Answer from the drawing. Dimensions are ordinates in mm from the lowest x, y and z of the part. Coordinates: 2 decimals unless noted, no trailing zeros. Loops run counter-clockwise (first coordinate to the right, second up) from the corner with the lowest first, then second, coordinate; pieces in that order, holes last. Notation, with made-up numbers: (33, -11) -> (60, -11) arc R33 cw to (60, 18) -> close; hole circle Ø9 at (-27.75, 38.5). An arc over 180 degrees is marked (long way). Use a Markdown table: item, result.
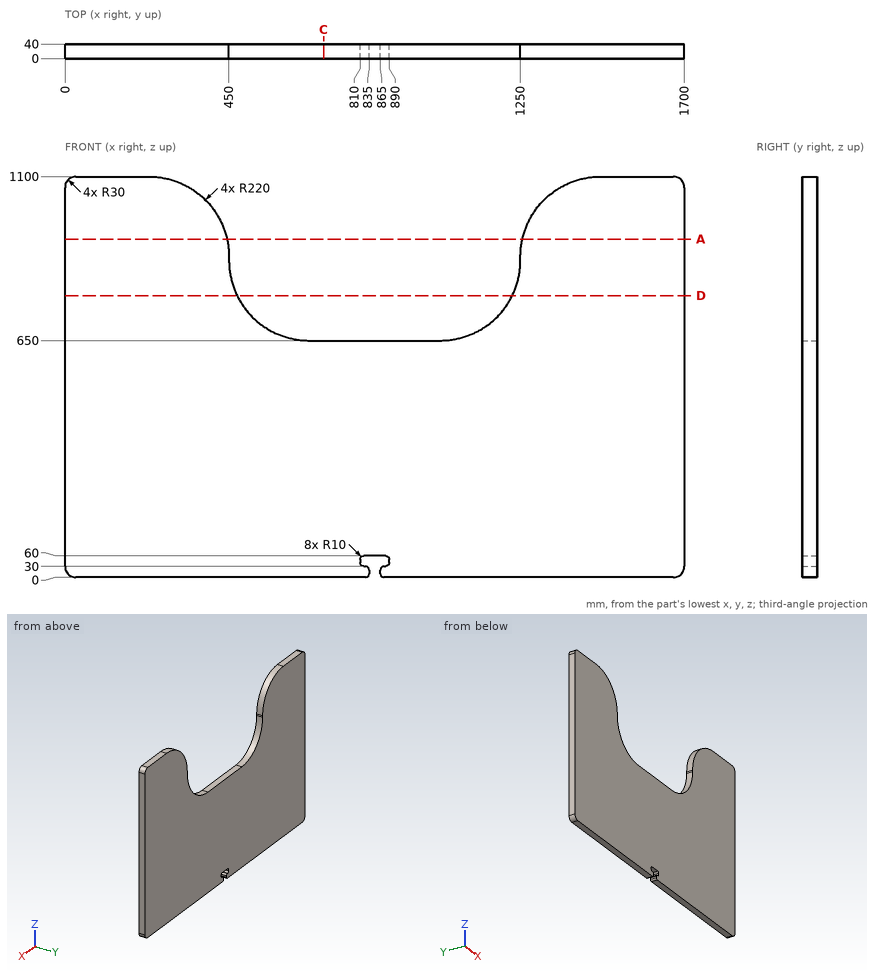
Q1. Section A-A on z = 928.5 is taken. Determine the outline of the cut face in (x, y).
Solved:
| item | result |
|---|---|
| outline | (0, 0) -> (444.59, 0) -> (444.59, 40) -> (0, 40) -> close; (1255.41, 0) -> (1700, 0) -> (1700, 40) -> (1255.41, 40) -> close |
Q2. Section C-C on x = 710 is taken. Determine the outline of the cut face in (y, z).
Solved:
| item | result |
|---|---|
| outline | (0, 0) -> (40, 0) -> (40, 650) -> (0, 650) -> close |
Q3. Section D-D on z = 773 is taken. Determine the outline of the cut face in (x, y).
Solved:
| item | result |
|---|---|
| outline | (0, 0) -> (472.54, 0) -> (472.54, 40) -> (0, 40) -> close; (1227.46, 0) -> (1700, 0) -> (1700, 40) -> (1227.46, 40) -> close |
Q4. Consider line 1 (X direction, y = 19.5, z = 774); line 2 (X direction, y = 30, z = 776); line 3 (Z direction, x = 758.5, y = 38). Determine where each line is inside the solid, lowest interval first. Write a range as [from, to].
Solved:
| item | result |
|---|---|
| line 1 | [0, 472.05], [1227.95, 1700] |
| line 2 | [0, 471.09], [1228.91, 1700] |
| line 3 | [0, 650] |
Q5. Given pin 1 Ø20 at (x, y) = (855, 21.5) entering from +Z; pin 2 Ø3 at (y, z) = (16.5, 14) entering from +X; pin 3 Ø4 at (x, y) = (522.5, 7) entering from +Z, each flat-ended and moving along its own axis, determine where each tip first touches the part or whether it passes through.
Solved:
| item | result |
|---|---|
| pin 1 | z = 650 |
| pin 2 | x = 1696.26 |
| pin 3 | z = 708.6 |
